Geometry: final body of the model. Coordinates: model frame, mm. A direction names the side the tool comes from. Round coordinates to 2 decimals unless told otherwise and drop trailing zeros. Write each loop counter-clockwise with the first axis right and the second up, starting at its lowest first coordinate (ties: lowest second). Pieces come first, ordered by that corner, then holes. Notation, with made-up numbers: (11, 44.5) -> (24, 44.5) arc R14 ccw to (24, 57.5) -> close; hole circle Ø9 at (14.25, -30). An arc over 180 degrees is marked (long way). One line per item, written item: value. Start each with the question number.
from build123d import *

# Parameters (mm, degrees)
SKETCH1_W               = 7
SKETCH1_H               = 5
SKETCH1_W_2             = 5.8
SKETCH1_H_2             = 3.8
BOSS_EXTRUDE1_DEPTH     = 2.8
SKETCH3_W               = 2.7
SKETCH3_H               = 8.95
SKETCH3_W_2             = 1.5
SKETCH3_H_2             = 7.75
BOSS_EXTRUDE2_DEPTH     = 2.7
SKETCH4_W               = 2.7
SKETCH4_H               = 4.55
BOSS_EXTRUDE3_DEPTH     = 0.6
SKETCH5_W               = 2.7
SKETCH5_H               = 8.95
BOSS_EXTRUDE4_DEPTH     = 0.6
SKETCH6_W               = 4.9
SKETCH6_H               = 5
BOSS_EXTRUDE5_DEPTH     = 0.6
FILLET2_R               = 0.7
SKETCH7_R               = 1
CUT_EXTRUDE1_DEPTH      = 1.7
SKETCH8_R               = 1.15
BOSS_EXTRUDE6_DEPTH     = 1.5
BOSS_EXTRUDE6_DRAFT     = -5
FILLET1_R               = 0.5
BOSS_EXTRUDE7_START     = -1.5
SKETCH8_2_R             = 1.15
BOSS_EXTRUDE7_DEPTH     = 1
BOSS_EXTRUDE7_DRAFT     = -10
CUT_EXTRUDE2_DEPTH      = 10.052209675
CUT_EXTRUDE2_DEPTH_BACK = 10.052209675
SKETCH9_R               = 0.75
FILLET3_R               = 0.5
FILLET5_R               = 0.5
FILLET6_R               = 0.5
FILLET7_R               = 0.5
CHAMFER1_SIZE           = 0.5


with BuildPart() as part:
    # Sketch1 → Boss-Extrude1 (new body)
    with BuildSketch(Plane(origin=(0, 0, 0), x_dir=(1, 0, 0), z_dir=(0, 1, 0))):
        Rectangle(SKETCH1_W, SKETCH1_H)
        Rectangle(SKETCH1_W_2, SKETCH1_H_2, mode=Mode.SUBTRACT)
    extrude(amount=BOSS_EXTRUDE1_DEPTH)

    # Sketch3 → Boss-Extrude2 (add)
    with BuildSketch(Plane(origin=(0, 2.8, 0), x_dir=(1, 0, 0), z_dir=(0, 1, 0))):
        with Locations((-2.15, -1.975)):
            Rectangle(SKETCH3_W, SKETCH3_H)
        with Locations((-2.15, -1.975)):
            Rectangle(SKETCH3_W_2, SKETCH3_H_2, mode=Mode.SUBTRACT)
    extrude(amount=BOSS_EXTRUDE2_DEPTH)

    # Sketch4 → Boss-Extrude3 (add)
    with BuildSketch(Plane.XZ.offset(-2.8)):
        with Locations((-2.15, 4.175)):
            Rectangle(SKETCH4_W, SKETCH4_H)
    extrude(amount=-BOSS_EXTRUDE3_DEPTH)

    # Sketch5 → Boss-Extrude4 (add)
    with BuildSketch(Plane(origin=(0, 5.5, 0), x_dir=(1, 0, 0), z_dir=(0, 1, 0))):
        with Locations((-2.15, -1.975)):
            Rectangle(SKETCH5_W, SKETCH5_H)
    extrude(amount=BOSS_EXTRUDE4_DEPTH)

    # Sketch6 → Boss-Extrude5 (add)
    with BuildSketch(Plane(origin=(0, 2.8, 0), x_dir=(1, 0, 0), z_dir=(0, 1, 0))):
        with Locations((1.05, 0)):
            Rectangle(SKETCH6_W, SKETCH6_H)
    extrude(amount=-BOSS_EXTRUDE5_DEPTH)

    # Fillet2
    fillet2_edges = [part.edges().sort_by_distance(p)[0] for p in [
        (-2.15, 5.5, -1.9),
        (-1.4, 5.5, 1.975),
        (-2.15, 5.5, 5.85),
        (-2.9, 5.5, 1.975),
    ]]
    fillet(fillet2_edges, radius=FILLET2_R)

    # Sketch7 → Cut-Extrude1 (cut)
    with BuildSketch(Plane.XZ.offset(-2.8)):
        with Locations(Location((-2.15, 4.85, 0), (0, 0, 270))):
            Circle(SKETCH7_R)
    extrude(amount=-CUT_EXTRUDE1_DEPTH, mode=Mode.SUBTRACT)


with BuildPart() as boss_extrude6_tool:
    # Sketch8 → Boss-Extrude6 (with draft: the straight prism first)
    with BuildSketch(Plane(origin=(0, 2.8, 0), x_dir=(-1, 0, 0), z_dir=(0, -1, 0))):
        with Locations((-1.5, 0)):
            Circle(SKETCH8_R)
    extrude(amount=-BOSS_EXTRUDE6_DEPTH)
    # Boss-Extrude6: the draft: its side faces are tilted about the plane it starts from
    boss_extrude6_sides = [boss_extrude6_tool.faces().sort_by_distance(p)[0] for p in [
        (2.65, 3.55, 0),
    ]]
    draft(boss_extrude6_sides, Plane(origin=(0, 2.8, 0), x_dir=(-1, 0, 0), z_dir=(0, -1, 0)), BOSS_EXTRUDE6_DRAFT)


with BuildPart() as part_1:
    add(part.part)

    # Boss-Extrude6: add boss_extrude6_tool
    add(boss_extrude6_tool.part)

    # Fillet1
    fillet1_edges = [part_1.edges().sort_by_distance(p)[0] for p in [
        (2.65, 2.8, 0),
    ]]
    fillet(fillet1_edges, radius=FILLET1_R)


with BuildPart() as boss_extrude7_tool:
    # Sketch8<2> → Boss-Extrude7 (with draft: the straight prism first)
    with BuildSketch(Plane(origin=(0, 2.8, 0), x_dir=(-1, 0, 0), z_dir=(0, -1, 0)).offset(BOSS_EXTRUDE7_START)):
        with Locations((-1.5, 0)):
            Circle(SKETCH8_2_R)
    extrude(amount=-BOSS_EXTRUDE7_DEPTH)
    # Boss-Extrude7: the draft: its side faces are tilted about the plane it starts from
    boss_extrude7_sides = [boss_extrude7_tool.faces().sort_by_distance(p)[0] for p in [
        (2.65, 4.8, 0),
    ]]
    draft(boss_extrude7_sides, Plane(origin=(0, 2.8, 0), x_dir=(-1, 0, 0), z_dir=(0, -1, 0)).offset(BOSS_EXTRUDE7_START), BOSS_EXTRUDE7_DRAFT)


with BuildPart() as part_2:
    add(part_1.part)

    # Boss-Extrude7: add boss_extrude7_tool
    add(boss_extrude7_tool.part)

    # Sketch9 → Cut-Extrude2 (cut, two sides: drawn at the far end of the back side and taken through both)
    with BuildSketch(Plane(origin=(0, 5.3, 0), x_dir=(1, 0, 0), z_dir=(0, 1, 0)).offset(-CUT_EXTRUDE2_DEPTH_BACK)):
        with Locations(Location((1.5, 0, 0), (0, 0, 90))):
            Circle(SKETCH9_R)
    extrude(amount=CUT_EXTRUDE2_DEPTH + CUT_EXTRUDE2_DEPTH_BACK, mode=Mode.SUBTRACT)

    # Fillet3
    fillet3_edges = [part_2.edges().sort_by_distance(p)[0] for p in [
        (-3.5, 6.1, 1.975),
        (-2.15, 6.1, 6.45),
        (-0.8, 6.1, 1.975),
        (-2.15, 6.1, -2.5),
    ]]
    fillet(fillet3_edges, radius=FILLET3_R)

    # Fillet5
    # the kernel refuses this fillet: 0.5 mm, written as the material it takes off along each edge
    with BuildSketch(Plane(origin=(-1.3, 5.6, -2), x_dir=(1, 0, 0), z_dir=(0, 0, -1))) as fillet5_piece_1_section:
        Polygon((0, 0), (FILLET5_R, 0), (FILLET5_R, -FILLET5_R), (0, -FILLET5_R), align=None)
    fillet5_piece_1 = extrude(amount=FILLET5_R, mode=Mode.PRIVATE)
    fillet5_piece_1 = fillet5_piece_1 - Plane(origin=(-1.3, 5.6, -2), x_dir=(-0.7071067811865475, -0.7071067811865475, 0), z_dir=(0, 0, -1)) * Sphere(FILLET5_R, mode=Mode.PRIVATE)
    add(fillet5_piece_1, mode=Mode.SUBTRACT)
    with BuildSketch(Plane(origin=(-1.3, 5.6, 5.95), x_dir=(0, 0, 1), z_dir=(1, 0, 0))) as fillet5_piece_2_section:
        Polygon((0, 0), (FILLET5_R, 0), (FILLET5_R, -FILLET5_R), (0, -FILLET5_R), align=None)
    fillet5_piece_2 = extrude(amount=FILLET5_R, mode=Mode.PRIVATE)
    fillet5_piece_2 = fillet5_piece_2 - Plane(origin=(-1.3, 5.6, 5.95), x_dir=(0, -0.7071067811865475, -0.7071067811865475), z_dir=(1, 0, 0)) * Sphere(FILLET5_R, mode=Mode.PRIVATE)
    add(fillet5_piece_2, mode=Mode.SUBTRACT)
    with BuildSketch(Plane(origin=(-3, 5.6, -2), x_dir=(-1, 0, 0), z_dir=(0, 0, -1))) as fillet5_piece_3_section:
        Polygon((0, 0), (FILLET5_R, 0), (FILLET5_R, FILLET5_R), (0, FILLET5_R), align=None)
    fillet5_piece_3 = extrude(amount=FILLET5_R, mode=Mode.PRIVATE)
    fillet5_piece_3 = fillet5_piece_3 - Plane(origin=(-3, 5.6, -2), x_dir=(0.7071067811865475, -0.7071067811865475, 0), z_dir=(0, 0, -1)) * Sphere(FILLET5_R, mode=Mode.PRIVATE)
    add(fillet5_piece_3, mode=Mode.SUBTRACT)
    with BuildSketch(Plane(origin=(-3, 5.6, 5.95), x_dir=(0, 0, 1), z_dir=(-1, 0, 0))) as fillet5_piece_4_section:
        Polygon((0, 0), (FILLET5_R, 0), (FILLET5_R, FILLET5_R), (0, FILLET5_R), align=None)
    fillet5_piece_4 = extrude(amount=FILLET5_R, mode=Mode.PRIVATE)
    fillet5_piece_4 = fillet5_piece_4 - Plane(origin=(-3, 5.6, 5.95), x_dir=(0, -0.7071067811865475, -0.7071067811865475), z_dir=(-1, 0, 0)) * Sphere(FILLET5_R, mode=Mode.PRIVATE)
    add(fillet5_piece_4, mode=Mode.SUBTRACT)
    with BuildSketch(Plane(origin=(-3.5, 1.55, 6.45), x_dir=(0, 0, -1), z_dir=(0, 1, 0)), Plane(origin=(-0.8, 5.6, 6.45), x_dir=(0, 0, -1), z_dir=(0, -1, 0)), Plane(origin=(-3.5, -1.25, 2.5), x_dir=(0, 0, -1), z_dir=(0, 1, 0))) as fillet5_piece_5:
        with BuildLine():
            CenterArc((FILLET5_R, -FILLET5_R), FILLET5_R, 90, 90)
            Line((0, -FILLET5_R), (0, 0))
            Line((0, 0), (FILLET5_R, 0))
        make_face()
    extrude(amount=4.05, mode=Mode.SUBTRACT)
    with BuildSketch(Plane(origin=(-3.5, -1.25, -2.5), x_dir=(1, 0, 0), z_dir=(0, 1, 0))) as fillet5_piece_6:
        with BuildLine():
            CenterArc((FILLET5_R, -FILLET5_R), FILLET5_R, 90, 90)
            Line((0, -FILLET5_R), (0, 0))
            Line((0, 0), (FILLET5_R, 0))
        make_face()
    extrude(amount=6.85, mode=Mode.SUBTRACT)
    with BuildSketch(Plane(origin=(-0.8, 5.6, -2.5), x_dir=(-1, 0, 0), z_dir=(0, -1, 0))) as fillet5_piece_7:
        with BuildLine():
            CenterArc((FILLET5_R, -FILLET5_R), FILLET5_R, 90, 90)
            Line((0, -FILLET5_R), (0, 0))
            Line((0, 0), (FILLET5_R, 0))
        make_face()
    extrude(amount=2.8, mode=Mode.SUBTRACT)
    with BuildSketch(Plane(origin=(3.5, 4.05, -2.5), x_dir=(-1, 0, 0), z_dir=(0, -1, 0)), Plane(origin=(3.5, 4.05, 2.5), x_dir=(0, 0, -1), z_dir=(0, -1, 0))) as fillet5_piece_8:
        with BuildLine():
            CenterArc((FILLET5_R, -FILLET5_R), FILLET5_R, 90, 90)
            Line((0, -FILLET5_R), (0, 0))
            Line((0, 0), (FILLET5_R, 0))
        make_face()
    extrude(amount=5.3, mode=Mode.SUBTRACT)

    # Fillet6
    # the kernel refuses this fillet: 0.5 mm, written as the material it adds along each edge
    with BuildSketch(Plane(origin=(-1.3, 2.8, -2), x_dir=(-0.5976672776328278, 0, 0.8017442392976482), z_dir=(0.8017442392976482, 0, 0.5976672776328278))) as fillet6_piece_1_section:
        with BuildLine():
            CenterArc((0.5 + FILLET6_R, -FILLET6_R), FILLET6_R, 90, 90)
            Line((0.5, -FILLET6_R), (0.5, 0))
            Line((0.5, 0), (0.5 + FILLET6_R, 0))
        make_face()
    fillet6_piece_1 = revolve(axis=Axis((-1.3, 2.8, -2), (0, -1, 0)), revolution_arc=233.296989237, mode=Mode.PRIVATE)
    fillet6_piece_1 = split(fillet6_piece_1, bisect_by=Plane(origin=(-0.925030534, 2.955814156, -2.5), z_dir=(0, 0, 1)), keep=Keep.TOP, mode=Mode.PRIVATE)
    fillet6_piece_1 = split(fillet6_piece_1, bisect_by=Plane(origin=(-0.925030534, 2.955814156, -1.9), z_dir=(0, 0, -1)), keep=Keep.TOP, mode=Mode.PRIVATE)
    add(fillet6_piece_1)
    with BuildSketch(Plane(origin=(-0.8, 2.8, 2.5), x_dir=(1, 0, 0), z_dir=(0, 0, -1))) as fillet6_piece_2:
        with BuildLine():
            CenterArc((FILLET6_R, -FILLET6_R), FILLET6_R, 90, 90)
            Line((0, -FILLET6_R), (0, 0))
            Line((0, 0), (FILLET6_R, 0))
        make_face()
    extrude(amount=4.5)

    # Fillet7
    # the kernel refuses this fillet: 0.5 mm, written as the material it adds along each edge
    with BuildSketch(Plane(origin=(-0.8, 2.8, 2.5), x_dir=(0, -1, 0), z_dir=(-1, 0, 0))) as fillet7_piece_1:
        with BuildLine():
            CenterArc((FILLET7_R, FILLET7_R), FILLET7_R, 180, 90)
            Line((0, FILLET7_R), (0, 0))
            Line((0, 0), (FILLET7_R, 0))
        make_face()
    extrude(amount=2.2)
    with BuildSketch(Plane(origin=(-3, 2.8, 2), x_dir=(0.8017442392976479, 0, -0.597667277632828), z_dir=(0.597667277632828, 0, 0.8017442392976479))) as fillet7_piece_2_section:
        with BuildLine():
            CenterArc((0.5 + FILLET7_R, -FILLET7_R), FILLET7_R, 90, 90)
            Line((0.5, -FILLET7_R), (0.5, 0))
            Line((0.5, 0), (0.5 + FILLET7_R, 0))
        make_face()
    fillet7_piece_2 = revolve(axis=Axis((-3, 2.8, 2), (0, 1, 0)), revolution_arc=233.296989237, mode=Mode.PRIVATE)
    fillet7_piece_2 = split(fillet7_piece_2, bisect_by=Plane(origin=(-3.5, 2.644185551, 2.37496936), z_dir=(1, 0, 0)), keep=Keep.TOP, mode=Mode.PRIVATE)
    fillet7_piece_2 = split(fillet7_piece_2, bisect_by=Plane(origin=(-2.9, 2.644185551, 2.37496936), z_dir=(-1, 0, 0)), keep=Keep.TOP, mode=Mode.PRIVATE)
    add(fillet7_piece_2)

    # Chamfer1
    chamfer1_edges = [part_2.edges().sort_by_distance(p)[0] for p in [
        (-2.15, 3.4, 1.9),
    ]]
    chamfer(chamfer1_edges, length=CHAMFER1_SIZE)


solid = part_2.part
(1) Pin query (flat end, axial travel): pin 1 (3 mm diameter, centred on x = 1.5, z = 1, fed in from +Y); pin 2 (2.5 mm diameter, centred on x = 1.5, z = 0, fed in from -Y). Return the tip coordinate at first contact, or that it passes through.
(2) Section query A-A (y = 4). Output: boundary loops of the cut face in (x, z).
(3) Pull-direction query (Z, two-part tool) for faces 4 (the face through (0, 1, 1.9)), 5 (the face through (3.5, 1, 0)), 6 (the face through (-2, 4, 6.45)), 7 (the face through (-2, 4, 5.85)); classes: pulls with the +Z half, pulls with the -Z half, needs draft (parallel to the pull), parting line crosses it, or undercut.
(4) Set-up query: faces 1 (the face through (-2.9, 3, 0)), 2 (the face through (-3.04, 3.45, 4.39)), 3 (the face through (0, 1, 2.5)). Return all of +Z, -Z, +X, -X, +Y, -Y with unobstructed straight access to the full face (end or side cutting, diameter ignored); none if empty.
(5) Section query B-B (z = 4.85). Output: boundary loops of the cut face in (x, y).
(6) Section query C-C (x = 1.5). Output: boundary loops of the cut face in (y, z), and give its area (3 significant figures).
(7) Line query: probe 1 along Z at (x, y) = (-2.15, 3.5); probe 2 along X at (y, z) = (3.65, 4.85); probe 3 along Z at (x, y) = (2, 2). Output: solid intervals per line, ascending.
(8) Section query D-D (y = 1.5). Output: boundary loops of the cut face in (x, z).
Results list:
1. pin 1: stops at y = 5.3
1. pin 2: stops at y = 2.2
2. outline: (-3.5, -2) arc R0.5 ccw to (-3, -2.5) -> (-1.3, -2.5) arc R0.5 ccw to (-0.8, -2) -> (-0.8, 5.95) arc R0.5 ccw to (-1.3, 6.45) -> (-3, 6.45) arc R0.5 ccw to (-3.5, 5.95) -> close; circle Ø2.09 at (1.5, 0); hole (-2.9, -1.9) -> (-1.4, -1.9) -> (-1.4, 4.19) arc R1 ccw to (-1.4, 5.51) -> (-1.4, 5.85) -> (-2.9, 5.85) -> (-2.9, 5.51) arc R1 ccw to (-2.9, 4.19) -> close; hole circle Ø1.5 at (1.5, 0)
3. face 4: undercut
3. face 5: needs draft
3. face 6: pulls with the +Z half
3. face 7: undercut
4. face 1: none
4. face 2: -Y
4. face 3: +Z, +X, -Y
5. outline: (-3.5, 2.8) -> (-3.15, 2.8) -> (-3.15, 4.5) -> (-2.9, 4.5) -> (-2.9, 4.8) arc R0.7 cw to (-2.2, 5.5) -> (-2.1, 5.5) arc R0.7 cw to (-1.4, 4.8) -> (-1.4, 4.5) -> (-1.15, 4.5) -> (-1.15, 2.8) -> (-0.8, 2.8) -> (-0.8, 5.6) arc R0.5 ccw to (-1.3, 6.1) -> (-3, 6.1) arc R0.5 ccw to (-3.5, 5.6) -> close
6. outline: (0, -2.5) -> (2.8, -2.5) -> (2.8, -1.61) arc R0.5 cw to (3.26, -1.11) -> (4.3, -1.02) -> (4.3, -1.15) -> (5.3, -0.97) -> (5.3, -0.75) -> (2.2, -0.75) -> (2.2, -1.9) -> (0, -1.9) -> close; (0, 1.9) -> (2.2, 1.9) -> (2.2, 0.75) -> (5.3, 0.75) -> (5.3, 0.97) -> (4.3, 1.15) -> (4.3, 1.02) -> (3.26, 1.11) arc R0.5 cw to (2.8, 1.61) -> (2.8, 2.5) -> (0, 2.5) -> close
6. area: 6.45 mm^2
7. probe 1: z = -2.5 to -1.9, 5.85 to 6.45
7. probe 2: x = -3.5 to -3.15, -1.15 to -0.8
7. probe 3: z = -2.5 to -1.9, 1.9 to 2.5
8. outline: (-3.5, -2) arc R0.5 ccw to (-3, -2.5) -> (3, -2.5) arc R0.5 ccw to (3.5, -2) -> (3.5, 2) arc R0.5 ccw to (3, 2.5) -> (-3, 2.5) arc R0.5 ccw to (-3.5, 2) -> close; hole (-2.9, -1.9) -> (2.9, -1.9) -> (2.9, 1.9) -> (-2.9, 1.9) -> close
